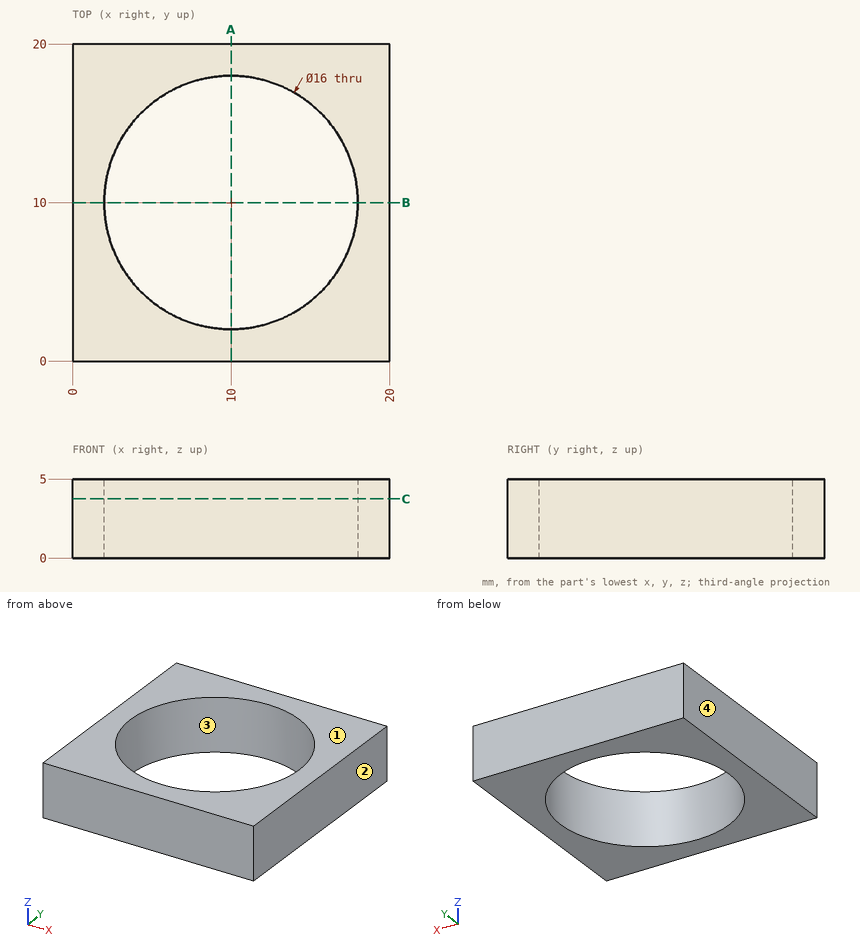
Drawing for the job (mm, zero at the part's lowest x, y, z). Give positions to 0.01 mm unless a question says otherwise; leave off trailing zeros. Loops run counter-clockwise (first coordinate to the right, second up) from the corner with the lowest first, then second, coordinate; pieces in that order, holes last.
1) Band-saw the part on A-A on x = 10. List the corners of the cut face in (y, z), then the cut area to 3 significant figures.
Values follow:
outline: (0, 0) - (2, 0) - (2, 5) - (0, 5) - close; (18, 0) - (20, 0) - (20, 5) - (18, 5) - close
area: 20.0 mm2
2) Drop a flat-ended pin along its axis: P1, Ø3, axis at x = 16, z = 4, coming from the -Y side. Give the stop position or say it passes through.
Values follow:
P1: stops at y = 0
3) Probe line 1 along X through (y, z) = (10, 2.9); line 2 along X through (y, z) = (16.25, 3.8). List the from-to ranges inside material, lowest first.
Values follow:
line 1: x = 0 to 2, 18 to 20
line 2: x = 0 to 5.01, 14.99 to 20
4) Two-plate mould, pull along X, no slides. Class the marked faces 1, 2, 3 and 4: released by +X, released by -X, zero draft, split by the parting line, or undercut.
Values follow:
face 1: zero draft
face 2: released by +X
face 3: undercut
face 4: released by -X
5) Band-saw the part on C-C on z = 3.75. List the corners of the cut face in (x, y).
Values follow:
outline: (0, 0) - (20, 0) - (20, 20) - (0, 20) - close; hole circle Ø16 at (10, 10)
